Autodesk Inventor part; units mm, degrees
ref_plane "YZ Plane" through (0, 0, 0) normal (1, 0, 0) x (0, 1, 0)
ref_plane "XZ Plane" through (0, 0, 0) normal (0, 1, 0) x (-1, 0, 0)
ref_plane "XY Plane" through (0, 0, 0) normal (0, 0, 1) x (1, 0, 0)
sketch "Sketch1" plane through (0, 0, 0) normal (0, 1, 0) x (-1, 0, 0)
  circle A0 centre (0, 0) radius 10
  dimension "d0" = 20
extrude "Extrusion1" add sketch "Sketch1" along normal blind 95
shell "Shell1" thickness 1 removed faces 0
sketch "Sketch3" plane through (0, 95, 0) normal (0, 1, 0) x (1, 0, 0)
  circle A0 centre (0, 0) radius 10
  line L0 (-3.1462, 1.4689) -> (3.1462, 1.4689)
  line L1 (4.1462, -0.5311) -> (4.1462, -1.4689)
  line L2 (4.1462, -1.4689) -> (-4.1462, -1.4689)
  line L3 (-4.1462, -1.4689) -> (-4.1462, -0.5311)
  line L4 (-4.1462, 1.4689) -> (4.1462, -1.4689) construction
  line L5 (4.1462, 1.4689) -> (-4.1462, -1.4689) construction
  line L6 (-4.1462, -0.5311) -> (-3.1462, 1.4689)
  line L7 (4.1462, -0.5311) -> (3.1462, 1.4689)
  dimension "d8" = 2
  dimension "d9" = 1
  dimension "d10" = 2
  dimension "d11" = 1
extrude "Extrusion3" cut sketch "Sketch3" against normal blind 5 contours L0 L7 L1 L2 L3 L6
properties part number "blank"
Could you check a few things on this model? Use its own coordinates, in mm. A direction names the side the tool comes from. Coordinates: 2 decimals unless noted, no trailing zeros. Order: outer loops, then holes, each group sorted by start corner. A loop starts at its lowest first (then second) coordinate and runs counter-clockwise, first axis right, second up. Notation, with made-up numbers: (-10, 27) -> (19, 27) arc R12 ccw to (19, 41) -> close; hole circle Ø6 at (-22.75, 28). An arc over 180 degrees is marked (long way). One line per question, with ' | ' between items.
Q1. Imagine slicing it at A-A on x = 0. Please give me the cut outline in (y, z).
Return value:
outline: (0, -10) -> (95, -10) -> (95, -1.47) -> (94, -1.47) -> (94, -9) -> (1, -9) -> (1, 9) -> (94, 9) -> (94, 1.47) -> (95, 1.47) -> (95, 10) -> (0, 10) -> close
Q2. I'm going to push flat-ended pins straight in: P1, Ø0.5, axis at y = 94.5, z = 1, coming from the +X side; P2, Ø1, axis at y = 94.5, z = 1, coming from the -X side; P3, Ø0.8, axis at x = 1, y = 94.5, coming from the -Z side. Where does each tip first touch, or does it pass through?
Return value:
P1: x = 9.97 | P2: x = -9.99 | P3: z = -9.98
Q3. Thinking about a two-plate mould opening in Z: for faces 3 (the face through (0, 0, 0)), 4 (the face through (0, 1, 0)), 5 (the face through (2.17, 46.84, 9.76)), which applies, pulls with the +Z half, pulls with the -Z half, needs draft (parallel to the pull), parting line crosses it, or undercut?
Return value:
face 3: needs draft | face 4: undercut | face 5: parting line crosses it
Q4. If I drill on L1, parallel to Y at x = 3.25, z = -5; L2, parallel to Z at x = 0, y = 27; L3, parallel to Z at x = 1, y = 23.5, over which ranges is the centre line in solid material (lowest first)?
Return value:
L1: 0 to 1, 94 to 95 | L2: -10 to -9, 9 to 10 | L3: -9.95 to -8.94, 8.94 to 9.95
Q5. Imagine slicing it at D-D on z = -3. Please give me the cut outline in (x, y).
Return value:
outline: (-9.54, 0) -> (9.54, 0) -> (9.54, 95) -> (-9.54, 95) -> close; hole (-8.49, 1) -> (8.49, 1) -> (8.49, 94) -> (-8.49, 94) -> close
Q6. Imagine slicing it at C-C on y = 14. Please give me the cut outline in (x, z), and give its area (3 significant figures).
Return value:
outline: circle Ø20 at (0, 0); hole circle Ø18 at (0, 0) | area: 59.7 mm²
Q7. Imagine slicing it at B-B on z = 6.25. Please give me the cut outline in (x, y), and give its area (3 significant figures).
Return value:
outline: (-7.81, 0) -> (7.81, 0) -> (7.81, 95) -> (-7.81, 95) -> close; hole (-6.48, 1) -> (6.48, 1) -> (6.48, 94) -> (-6.48, 94) -> close | area: 279 mm²
Q8. On a 3-axis mill with a long thin cutter (end or side, diameter ignored), from which of +Z, -Z, +X, -X, +Y, -Y can I reach the whole of each face in a straight line? I mean faces 1 (the face through (0, 95, -2)), 2 (the face through (0, 94, -2)). Say none if no direction works.
Return value:
face 1: +Z, -Z, +X, -X, +Y | face 2: none
